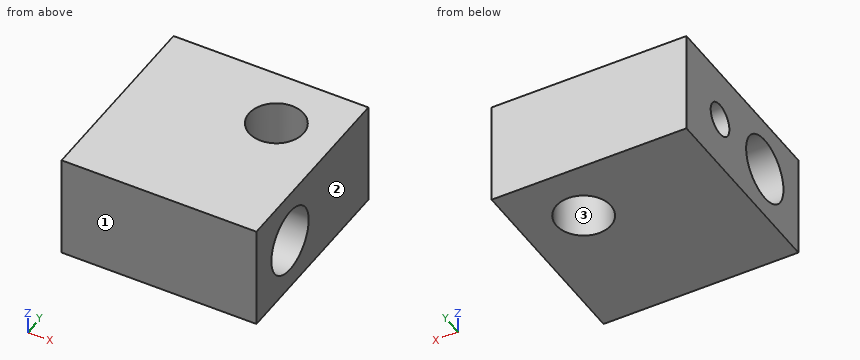
```python
from build123d import *

# Parameters (mm, degrees)
SKETCH1_W                      = 15
SKETCH1_H                      = 15
BOSS_EXTRUDE1_DEPTH            = 8
TAP_DRILL_FOR_M5X0_8_TAP1_D    = 4.2
F_5_0_5_DIAMETER_HOLE1_D       = 5
F_2_5_2_5_DIAMETER_HOLE1_D     = 2.5
F_2_5_2_5_DIAMETER_HOLE1_DEPTH = 6.05
F_2_5_2_5_DIAMETER_HOLE1_TIP   = 0.751075774


with BuildPart() as part:
    # Sketch1 → Boss-Extrude1 (new body)
    with BuildSketch(Plane.XY):
        with Locations((7.5, 7.5)):
            Rectangle(SKETCH1_W, SKETCH1_H)
    extrude(amount=BOSS_EXTRUDE1_DEPTH)

    # Tap Drill for M5x0.8 Tap1 (through all)
    with Locations(Plane.XY.offset(8)):
        with Locations((10.5, 10.5)):
            Hole(TAP_DRILL_FOR_M5X0_8_TAP1_D / 2)

    # Ø5.0 (5) Diameter Hole1 (through all)
    with Locations(Plane.ZY):
        with Locations((4, 4.5)):
            Hole(F_5_0_5_DIAMETER_HOLE1_D / 2)

    # Ø2.5 (2.5) Diameter Hole1
    with Locations(Plane.ZY):
        with Locations((4, 10.5)):
            Hole(F_2_5_2_5_DIAMETER_HOLE1_D / 2, depth=F_2_5_2_5_DIAMETER_HOLE1_DEPTH)
            with Locations((0, 0, -(F_2_5_2_5_DIAMETER_HOLE1_DEPTH + F_2_5_2_5_DIAMETER_HOLE1_TIP / 2))):  # 118° drill point
                Cone(0, F_2_5_2_5_DIAMETER_HOLE1_D / 2, F_2_5_2_5_DIAMETER_HOLE1_TIP, mode=Mode.SUBTRACT)


solid = part.part
```
Geometry check sheet. Reference: the model listing, model coordinates, mm. Face numbers are marked on the shaded views. Coordinates: 2 decimals unless noted, no trailing zeros. Order: outer loops, then holes, each group sorted by start corner. A loop starts at its lowest first (then second) coordinate and runs counter-clockwise, first axis right, second up. Notation, with made-up numbers: (8, -33) - (12, -33) arc R19 cw to (12, -16) - close; hole circle Ø3 at (33.25, 36). An arc over 180 degrees is marked (long way). Answer as a JSON object with one key per item and string values. Group by question number.
Item 1: Draft check along X on the marked faces 1, 2 and 3. Enter one of: +X half, -X half, draft (parallel to the pull), parting line (faces both ways), or undercut.
Item 2: Sectioned sample at B-B, the plane x = 9.75. Record the cut outline in (y, z), and give its area (3 significant figures).
Item 3: Scan lines: probe 1 along Y at (x, z) = (2.5, 4); probe 2 along Y at (x, z) = (10.5, 4); probe 3 along Z at (x, y) = (2, 10.5). Record each from-to range of solid material in increasing order.
Item 4: Sectioned sample at C-C, the plane y = 5. Record the cut outline in (x, z).
Item 5: Sectioned sample at A-A, the plane z = 2.5. Record the cut outline in (x, y), and give its area (3 significant figures).
Item 6: Sectioned sample at D-D, the plane z = 7.75. Record the cut outline in (x, y).
Resolved:
{
 "1": {"face 1": "draft", "face 2": "+X half", "face 3": "undercut"},
 "2": {"outline": "(0, 0) - (8.54, 0) - (8.54, 8) - (0, 8) - close; (12.46, 0) - (15, 0) - (15, 8) - (12.46, 8) - close; hole circle Ø5 at (4.5, 4)", "area": "69.0 mm^2"},
 "3": {"probe 1": "0 to 2, 7 to 9.25, 11.75 to 15", "probe 2": "0 to 2, 7 to 8.4, 12.6 to 15", "probe 3": "0 to 2.75, 5.25 to 8"},
 "4": {"outline": "(0, 0) - (15, 0) - (15, 1.55) - (0, 1.55) - close; (0, 6.45) - (15, 6.45) - (15, 8) - (0, 8) - close"},
 "5": {"outline": "(0, 0) - (15, 0) - (15, 2.5) - (0, 2.5) - close; (0, 6.5) - (15, 6.5) - (15, 15) - (0, 15) - close; hole circle Ø4.2 at (10.5, 10.5)", "area": "151 mm^2"},
 "6": {"outline": "(0, 0) - (15, 0) - (15, 15) - (0, 15) - close; hole circle Ø4.2 at (10.5, 10.5)"}
}
